Autodesk Inventor part; units mm, degrees
ref_plane "YZ Plane" through (0, 0, 0) normal (1, 0, 0) x (0, 1, 0)
ref_plane "XZ Plane" through (0, 0, 0) normal (0, 1, 0) x (-1, 0, 0)
ref_plane "XY Plane" through (0, 0, 0) normal (0, 0, 1) x (1, 0, 0)
sketch "Sketch1" plane through (0, 0, 0) normal (0, 1, 0) x (-1, 0, 0)
  line L0 (-12.5, 12.5) -> (12.5, 12.5)
  line L1 (12.5, 12.5) -> (12.5, -12.5)
  line L2 (12.5, -12.5) -> (-12.5, -12.5)
  line L3 (-12.5, -12.5) -> (-12.5, 12.5)
  line L4 (-12.5, 12.5) -> (12.5, -12.5)
  line L5 (12.5, 12.5) -> (-12.5, -12.5) construction
  point P0 (0, 0)
  point P1 (0, 0)
  point P2 (0, 0)
  dimension "d0" = 25
extrude "Extrusion1" add sketch "Sketch1" along normal blind 20 contours L0 L1 L4
sketch "Sketch2" plane through (0, 20, 0) normal (0, 1, 0) x (1, 0, 0)
  line L0 (9.5, 9.5) -> (-9.5, 9.5)
  line L1 (-9.5, 9.5) -> (-9.5, -9.5)
  line L2 (-9.5, -9.5) -> (9.5, -9.5)
  line L3 (9.5, -9.5) -> (9.5, 9.5)
  line L4 (9.5, 9.5) -> (-9.5, -9.5) construction
  line L5 (-9.5, 9.5) -> (9.5, -9.5) construction
  line L6 (-12.5, 12.5) -> (-12.5, -12.5)
  line L7 (-12.5, -12.5) -> (12.5, -12.5)
  point P0 (0, 0)
  dimension "d3" = 3
  dimension "d4" = 3
extrude "Extrusion2" cut sketch "Sketch2" against normal blind 17
sketch "Sketch5" plane through (-12.5, 0, 12.5) normal (0, 0, 1) x (1, 0, 0)
  line L0 (0, 0) -> (0, 20) construction
  line L1 (0, 10) -> (25, 10) construction
  line L2 (25, 8) -> (0, 8)
  line L3 (0, 8) -> (0, 12)
  line L4 (0, 12) -> (25, 12)
  line L5 (25, 12) -> (25, 8)
  line L6 (25, 8) -> (0, 12) construction
  line L7 (0, 8) -> (25, 12) construction
  line L8 (25, 0) -> (25, 20)
  point P0 (12.5, 0)
  point P1 (12.5, 10)
  dimension "d22" = 4
extrude "Extrusion5" add sketch "Sketch5" along normal blind 1
sketch "Sketch6" plane through (-12.5, 0, -12.5) normal (-1, 0, 0) x (0, 0, 1)
  line L0 (25, 8) -> (26, 8)
  line L1 (26, 8) -> (0, 8)
  line L2 (0, 8) -> (0, 12)
  line L3 (0, 12) -> (26, 12)
  line L4 (26, 12) -> (26, 8)
  line L5 (0, 0) -> (0, 20)
  point P0 (12.5, 0)
extrude "Extrusion6" add sketch "Sketch6" along normal blind 1
chamfer "Chamfer4" distance 1 angle 45 4 edges at (-12.5, 12, 0) (0, 12, 12.5) (0, 8, 12.5) (-12.5, 8, 0)
sketch "Sketch7" plane through (9.5, 20, 9.5) normal (0, 0, -1) x (-1, 0, 0)
  line L0 (19, 0) -> (19, -17) construction
  line L1 (23, -12) -> (23, -8)
  line L2 (23, -10) -> (-3, -10) construction
  line L3 (9.5, -20) -> (9.5, 0) construction
  line L4 (0, 0) -> (19, 0)
  circle A0 centre (9.5, -10) radius 1.7
  dimension "d30" = 3.4
extrude "Extrusion7" cut sketch "Sketch7" against normal through all
sketch "Sketch8" plane through (-9.5, 20, 9.5) normal (1, 0, 0) x (0, 0, -1)
  line L0 (9.5, -20) -> (9.5, 0) construction
  line L1 (0, 0) -> (19, 0)
  line L2 (-1.6609, -10) -> (22, -10) construction
  line L3 (22, -13) -> (22, -7)
  circle A0 centre (9.5, -10) radius 1.7
  dimension "d33" = 3.4
extrude "Extrusion8" cut sketch "Sketch8" against normal through all
chamfer "Chamfer5" distance 1 angle 45 2 edges at (12.5, 10, 13.5) (-13.5, 10, -12.5)
chamfer "Chamfer6" distance 2 angle 45 3 edges at (-9.5, 11.5, 9.5) (-9.5, 3, 0) (0, 3, 9.5)
chamfer "Chamfer7" distance 0.5 angle 45 5 edges at (-12.5, 0, 0) (0, 0, 12.5) (0, 0, 0) (-12.5, 20, 0) (0, 20, 12.5)
properties part number "Corner Bracket" material "ABS Plastic"
Geometry check sheet. Reference: the model listing, model coordinates, mm. A direction names the side the tool comes from. Give positions to 0.01 mm unless a question says otherwise; leave off trailing zeros. Write each loop counter-clockwise with the first axis right and the second up, starting at its lowest first coordinate (ties: lowest second). Pieces come first, ordered by that corner, then holes. Notation, with made-up numbers: M -38,74 L -16,74 A25 cw -16,100 Z; hole C 35.25,85 d7. An arc over 180 degrees is marked long. Answer as CSV lines item,"result". Start each with the question number.
Q1. Section check A-A, the plane y = 10. Give the number of separate pieces and of enclosed holes in the cut face, then the cut area to 3 significant figures.
Q2. Material ranges on L1, parallel to Y at x = -10.55, z = 0; L2, parallel to Z at x = 1.75, y = 5; L3, parallel to Z at x = -11.5, y = 2.5, recorded low to high.
Q3. Go/stop test with flat-tipped pins: pin 1 (2 mm diameter, centred on y = 16.5, z = 6, fed in from -X); pin 2 (3.5 mm diameter, centred on x = 5, y = 5, fed in from +Z); pin 3 (7.5 mm diameter, centred on x = -2.5, z = 1.5, fed in from +Y); pin 4 (2 mm diameter, centred on x = 3, z = 8.5, fed in from -Y). Record where each tip stops, or that it passes through.
Q4. Tool access check on faces 1 (the face through (0, 16, 12.5)), 2 (the face through (0, 4, 12.5)), 3 (the face through (1, 13, 9.5)). Record the directions out of +Z, -Z, +X, -X, +Y, -Y that give a thin tool (end or side, any length) a straight path to the whole face; none if there is none.
Q5. Section check D-D, the plane y = 5.75. Record the cut outline in (x, z).
Q6. Release check for a two-part mould opening along Z. For faces 4 (the face through (-0.3, 12.5, 13)), 5 (the face through (-11.47, 8.34, 0.37)), 6 (the face through (-12.5, 4, 0)) record: pulls with the +Z half, pulls with the -Z half, needs draft (parallel to the pull), parting line crosses it, or undercut.
Geometry says:
1,separate pieces,"3"
1,enclosed holes,"0"
1,area,"157 mm^2"
2,L1,"0 to 8.3, 11.7 to 20"
2,L2,"9.5 to 12.5"
2,L3,"-11.5 to 12.5"
3,pin 1,"x = -12.5"
3,pin 2,"z = 12.5"
3,pin 3,"y = 3"
3,pin 4,"y = 0"
4,face 1,"+Z, +X, -X, +Y"
4,face 2,"+Z, +X, -X, -Y"
4,face 3,"-Z, +X, +Y"
5,outline,"M -12.5,-12.5 L -9.5,-9.5 L -9.5,7.5 L -7.5,9.5 L 9.5,9.5 L 12.5,12.5 L -12.5,12.5 Z"
6,face 4,"pulls with the +Z half"
6,face 5,"undercut"
6,face 6,"needs draft"
